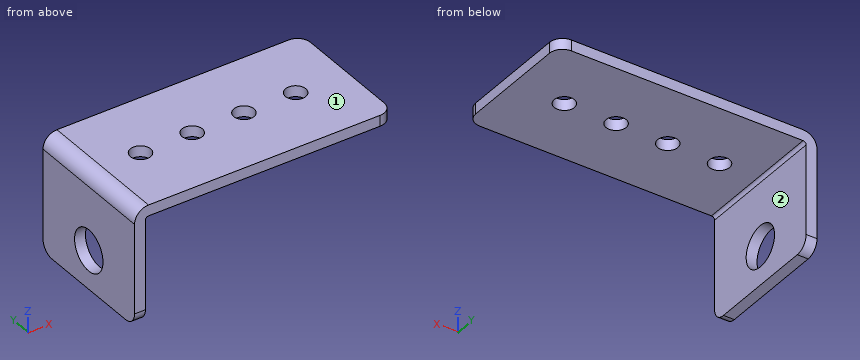
from build123d import *

# Parameters (mm, degrees)
BASE_FLANGE1_DEPTH = 32.766
SKETCH6_R          = 2.4892
CUT_EXTRUDE1_DEPTH = 77.00713927
SKETCH7_R          = 5.08
CUT_EXTRUDE2_DEPTH = 75.771620753
FILLET1_R          = 3.175


# Read off the part's stored shape, not the designer's step: Base-Flange1
with BuildPart() as part:
    # Base-Flange1 outline → Base-Flange1 (new body)
    with BuildSketch(Plane(origin=(0, 0, 0), x_dir=(1, 0, 0), z_dir=(0, 1, 0))):
        with BuildLine():
            Line((3.429, 0), (63.5, 0))
            Line((63.5, 0), (63.5, 2.667))
            Line((63.5, 2.667), (3.429, 2.667))
            ThreePointArc((3.429, 2.667), (2.890184633, 2.890184633), (2.667, 3.429))
            Line((2.667, 3.429), (2.667, 28.575))
            Line((2.667, 28.575), (0, 28.575))
            Line((0, 28.575), (0, 3.429))
            ThreePointArc((0, 3.429), (1.004330847, 1.004330847), (3.429, 0))
        make_face()
    extrude(amount=BASE_FLANGE1_DEPTH)

    # Sketch6 → Cut-Extrude1 (cut, through all)
    with BuildSketch(Plane(origin=(0, 0, -2.667), x_dir=(-1, 0, 0), z_dir=(0, 0, -1))):
        with Locations((-50.8, 16.383)):
            Circle(SKETCH6_R)
        with Locations((-38.1, 16.383)):
            Circle(SKETCH6_R)
        with Locations((-25.4, 16.383)):
            Circle(SKETCH6_R)
        with Locations((-12.7, 16.383)):
            Circle(SKETCH6_R)
    extrude(amount=-CUT_EXTRUDE1_DEPTH, mode=Mode.SUBTRACT)

    # Sketch7 → Cut-Extrude2 (cut, through all)
    with BuildSketch(Plane(origin=(2.667, 0, 0), x_dir=(0, 0, -1), z_dir=(1, 0, 0))):
        with Locations((19.05, 16.383)):
            Circle(SKETCH7_R)
    extrude(amount=-CUT_EXTRUDE2_DEPTH, mode=Mode.SUBTRACT)

    # Fillet1
    fillet1_edges = [part.edges().sort_by_distance(p)[0] for p in [
        (1.3335, 32.766, -28.575),
        (1.3335, 0, -28.575),
        (63.5, 32.766, -1.3335),
        (63.5, 0, -1.3335),
    ]]
    fillet(fillet1_edges, radius=FILLET1_R)


solid = part.part
Work out the finished part from the listing and answer in its coordinate system (mm). Face numbers are marked on the shaded views. A direction names the side the tool comes from. Round coordinates to 2 decimals unless told otherwise and drop trailing zeros. Write each loop counter-clockwise with the first axis right and the second up, starting at its lowest first coordinate (ties: lowest second). Pieces come first, ordered by that corner, then holes.
1) A cutting plane is placed at D-D (y = 15). Give the vertices of the cut face in (x, z) (3 decimals).
2) Given pin 1 Ø13 at (y, z) = (16.383, -19.05) entering from +X; pin 2 Ø3 at (x, y) = (16.5, 13.5) entering from -Z, each flat-ended and moving along its own axis, determine where each tip first touches the part or whether it passes through.
3) A tool of negligible diameter and unlimited length cuts with its end or side. For the marked faces 1 and 2, from which of +Z, -Z, +X, -X, +Y, -Y can it reach the whole face along a straight path? Write none if from no direction.
4) Straight lines are drawn through the part: line 1 (Y direction, x = 12.7, z = -1.75); line 2 (Z direction, x = 10, y = 19); line 3 (Y direction, x = 2.15, z = -19.05). For each, find the intervals that lie inside material, in ascending order.
5) A cutting plane is placed at C-C (y = 27.5). Give the vertices of the cut face in (x, z) (3 decimals), plus the area to 3 significant figures.
6) A cutting plane is placed at A-A (x = 50.8). Give the vertices of the cut face in (y, z), plus the area to 3 significant figures.
7) A cutting plane is placed at B-B (z = -19.05). Give the vertices of the cut face in (x, y), plus the area to 3 significant figures.
Completed:
1. outline: (0, -28.575) - (2.667, -28.575) - (2.667, -23.938) - (0, -23.938) - close; (0, -14.162) - (2.667, -14.162) - (2.667, -3.429) arc R0.762 cw to (3.429, -2.667) - (10.63, -2.667) - (10.63, 0) - (3.429, 0) arc R3.429 ccw to (0, -3.429) - close; (14.77, -2.667) - (23.33, -2.667) - (23.33, 0) - (14.77, 0) - close; (27.47, -2.667) - (36.03, -2.667) - (36.03, 0) - (27.47, 0) - close; (40.17, -2.667) - (48.73, -2.667) - (48.73, 0) - (40.17, 0) - close; (52.87, -2.667) - (63.5, -2.667) - (63.5, 0) - (52.87, 0) - close
2. pin 1: stops at x = 2.67
2. pin 2: stops at z = -2.67
3. face 1: +Z, +X, -X, +Y, -Y
3. face 2: -Z, +X, +Y, -Y
4. line 1: y = 0 to 13.89, 18.87 to 32.77
4. line 2: z = -2.67 to 0
4. line 3: y = 0 to 11.3, 21.46 to 32.77
5. outline: (0, -28.575) - (2.667, -28.575) - (2.667, -3.429) arc R0.762 cw to (3.429, -2.667) - (63.5, -2.667) - (63.5, 0) - (3.429, 0) arc R3.429 ccw to (0, -3.429) - close
5. area: 236 mm2
6. outline: (0, -2.67) - (13.89, -2.67) - (13.89, 0) - (0, 0) - close; (18.87, -2.67) - (32.77, -2.67) - (32.77, 0) - (18.87, 0) - close
6. area: 74.1 mm2
7. outline: (0, 0) - (2.67, 0) - (2.67, 11.3) - (0, 11.3) - close; (0, 21.46) - (2.67, 21.46) - (2.67, 32.77) - (0, 32.77) - close
7. area: 60.3 mm2
